Here's how the part is built. I have some questions about the finished solid (model axes, mm). Round coordinates to 2 decimals unless told otherwise and drop trailing zeros. Write each loop counter-clockwise with the first axis right and the second up, starting at its lowest first coordinate (ties: lowest second). Pieces come first, ordered by that corner, then holes. Notation, with made-up numbers: (15, 2) - (19, 2) arc R9 ccw to (19, 10) - close; hole circle Ø2 at (79, 34.5). An arc over 180 degrees is marked (long way). One line per question, with ' | ' between items. Start each with the question number.
(1) Imagine slicing it at A-A (x = 4.25). Write out the boundary of the cut face in (y, z), plus the area to 3 significant figures.
(2) Will these pins go through, and if not, where does the flat tip stop? pin 1 (3 mm diameter, centred on x = 5, y = 0.5, fed in from -Z); pin 2 (2 mm diameter, centred on y = 1.5, z = 1, fed in from -X); pin 3 (1 mm diameter, centred on x = 4, z = -1, fed in from +Y).
(3) Thinking about a two-plate mould opening in Y: for faces 1 (the flat face through (2.1, -1.2, -1.2)), 2 (the cylindrical face through (6.04, -1.5, 0.07)), 3 (the conical face through (1.87, -0.02, -0.02)), which applies, pulls with the +Y half, pulls with the -Y half, needs draft (parallel to the pull), parting line crosses it, or undercut?
(4) Imagine slicing it at C-C (y = 2.4). Write out the boundary of the cut face in (x, z), plus the area to 3 significant figures.
(5) Imagine slicing it at B-B (y = -2.15). Write out the boundary of the cut face in (x, z), plus the area to 3 significant figures.
(6) If I drill on L1, parallel to Z at x = 2, y = 0.95; L2, parallel to Z at x = 2.5, y = -0.85; L3, parallel to Y at x = 1.25, z = 0.7 (3 decimals), over which ranges is the centre line in solid material (lowest first)?
from build123d import *

# Parameters (mm, degrees)
SKETCH3_W    = 0.53
SKETCH3_H    = 3
SKETCH4_W    = 0.53
SKETCH4_H    = 1.304822816
RECPAT_COUNT = 2
RECPAT_ANGLE = 90


with BuildPart() as part:
    # BodySke → Base-Revolve (revolve)
    with BuildSketch(Plane.XY):
        with BuildLine():
            Line((2.1, 1.5), (2.1, 2.787471973))
            ThreePointArc((2.1, 2.787471973), (0.583753036, 1.744992837), (0, 0))
            Line((0, 0), (10.1, 0))
            Line((10.1, 0), (10.1, 1.5))
            Line((10.1, 1.5), (2.1, 1.5))
        make_face()
    revolve(axis=Axis((-25.4, 0, 0), (1, 0, 0)))

    # Sketch3 → Recess section 0
    with BuildSketch(Plane(origin=(0, 0, 0), x_dir=(0, 0, -1), z_dir=(1, 0, 0))):
        Rectangle(SKETCH3_W, SKETCH3_H)
    # Sketch4 → Recess section 1
    with BuildSketch(Plane(origin=(1.7, 0, 0), x_dir=(0, 0, -1), z_dir=(1, 0, 0))):
        Rectangle(SKETCH4_W, SKETCH4_H)
    recess = loft(mode=Mode.SUBTRACT)

    # RecPat: Recess ×2 about axis
    recpat_axis = Axis((0, 0, 0), (1, 0, 0))
    for i in range(1, RECPAT_COUNT):
        add(recess.rotate(recpat_axis, i * RECPAT_ANGLE / (RECPAT_COUNT - 1)), mode=Mode.SUBTRACT)

    # RecCorSke → RecessCore (revolve, cut)
    with BuildSketch(Plane.XY):
        Polygon((0, 0), (0, 0.67487558), (1.7, 0.556), (1.880655351, 0), align=None)
    revolve(axis=Axis((-3.175, 0, 0), (1, 0, 0)), mode=Mode.SUBTRACT)


solid = part.part
Check sheet entries:
1) outline: circle Ø3 at (0, 0) | area: 7.07 mm^2
2) pin 1: z = -1.5 | pin 2: x = 0.11 | pin 3: y = 1.41
3) face 1: needs draft | face 2: parting line crosses it | face 3: undercut
4) outline: (2.1, -1.42) - (2.1, 1.42) arc R1.63 ccw to start | area: 1.67 mm^2
5) outline: (2.1, -1.77) - (2.1, 1.77) arc R1.95 ccw to start | area: 2.93 mm^2
6) L1: -2.59 to 2.59 | L2: -1.24 to 1.24 | L3: -2.28 to -0.265, 0.265 to 2.28
